```python
from build123d import *


with BuildPart() as part:
    # Esboço1 → Revolução1 (revolve)
    with BuildSketch(Plane.XY, mode=Mode.PRIVATE) as revolu_o1_sk:
        Polygon((0.465967208, 5.756230657), (2.565967208, 5.756230657), (3.000371133, 6.797789179), (8.065967208, 6.797789179), (8.065967208, 7.047789179), (40.765967208, 7.362789179), (40.765967208, 7.047789179), (40.765967208, 6.662789179), (8.765967208, 6.347789179), (8.765967208, 6.097789179), (7.343223511, 6.097789179), (3.466863641, 6.097789179), (2.910073766, 4.762789179), (2.246620738, 4.762789179), (0.88387569, 4.762789179), (0.88387569, 5.112789179), (2.246620738, 5.112789179), (2.246620738, 5.406230657), (0.465967208, 5.406230657), align=None)
    revolve(revolu_o1_sk.sketch.rotate(Axis((0.88387569, 3.587789179, 0), (1, 0, 0)), 90), axis=Axis((0.88387569, 3.587789179, 0), (1, 0, 0)))


solid = part.part
```
Check sheet for the modelled part. Datum: model origin and axes. Units: mm. A direction names the side the tool comes from. Coordinates: 2 decimals unless noted, no trailing zeros. Loops run counter-clockwise (first coordinate to the right, second up) from the corner with the lowest first, then second, coordinate; pieces in that order, holes last.
1) Material ranges on probe 1 along Y at (x, z) = (1.95, 0); probe 2 along X at (y, z) = (6.75, -1); probe 3 along Z at (x, y) = (9.5, 5.25), recorded low to high.
2) Release check for a two-part mould opening along Y. For faces 1 (the face through (5.57, 6.72, -0.7)), 2 (the face through (1.575, 5.077, -0.331)), 3 (the face through (40.766, 7, -1)) record: released by +Y, released by -Y, zero draft, split by the parting line, or undercut.
3) Access from +Z, -Z, +X, -X, +Y, -Y to the whole of each face (thin tool, end or side, straight path). Record for faces 4 (the face through (24.5, 0.7, -0.4)), 5 (the face through (24.64, 6.8, 1.67)), 6 (the face through (1.911, 4.735, -0.255)).
4) Sectioned sample at B-B (x = 30). Record the boundary of the cut face in (y, z).
5) Gauge pin test, flat ends, axial feed: pin 1 (2 mm diameter, centred on x = 20.5, y = 3.5, fed in from +Z); pin 2 (1.1 mm diameter, centred on y = 3, z = 0.5, fed in from -X); pin 3 (1.5 mm diameter, centred on x = 24, z = -0.5, fed in from +Y); pin 4 (2.5 mm diameter, centred on y = 4, z = 0.5, fed in from -X). Record the tip position at first contact, or that the pin passes through.
6) Sectioned sample at A-A (x = 23). Record the boundary of the cut face in (y, z), and give its area (3 significant figures).
Check sheet entries:
1. probe 1: y = 1.42 to 1.77, 2.06 to 2.41, 4.76 to 5.11, 5.41 to 5.76
1. probe 2: x = 8.07 to 40.77
1. probe 3: z = -3.05 to -2.21, 2.21 to 3.05
2. face 1: split by the parting line
2. face 2: undercut
2. face 3: zero draft
3. face 4: +X
3. face 5: -X
3. face 6: +X, -X
4. outline: circle Ø7.34 at (3.59, 0); hole circle Ø5.94 at (3.59, 0)
5. pin 1: stops at z = 3.59
5. pin 2: stops at x = 0.88
5. pin 3: stops at y = 7.21
5. pin 4: stops at x = 0.47
6. outline: circle Ø7.21 at (3.59, 0); hole circle Ø5.8 at (3.59, 0)
6. area: 14.4 mm2
